from build123d import *

# Parameters (mm, degrees)
F0_R     = 22
F0_R_2   = 17.5
F0_R_3   = 12
F1_DEPTH = 8
F2_DEPTH = 20
F3_R     = 3
F4_R     = 1
F5_R     = 1


with BuildPart() as f1:
    # F0 (on Front) → F1 (new body)
    with BuildSketch(Plane.XZ):
        Circle(F0_R)
        Circle(F0_R_2, mode=Mode.SUBTRACT)
        Circle(F0_R_2)
        Circle(F0_R_3, mode=Mode.SUBTRACT)
    extrude(amount=F1_DEPTH)

    # F0 (on Front) → F2 (join)
    with BuildSketch(Plane.XZ):
        Circle(F0_R_2)
        Circle(F0_R_3, mode=Mode.SUBTRACT)
    extrude(amount=F2_DEPTH)

    # F3
    f3_edges = [f1.edges().sort_by_distance(p)[0] for p in [
        (-22, 0, 0),
    ]]
    fillet(f3_edges, radius=F3_R)

    # F4
    f4_edges = [f1.edges().sort_by_distance(p)[0] for p in [
        (-22, -8, 0),
    ]]
    fillet(f4_edges, radius=F4_R)

    # F5
    f5_edges = [f1.edges().sort_by_distance(p)[0] for p in [
        (-17.5, -20, 0),
    ]]
    fillet(f5_edges, radius=F5_R)


solid = f1.part
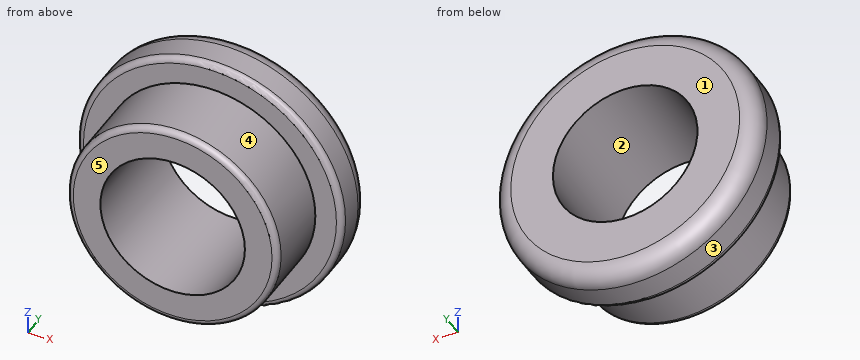
Source: CAD feature listing. Evaluate the final solid. Frame: model axes, mm. Face numbers are marked on the shaded views. A direction names the side the tool comes from. Round coordinates to 2 decimals unless told otherwise and drop trailing zeros. Loops run counter-clockwise (first coordinate to the right, second up) from the corner with the lowest first, then second, coordinate; pieces in that order, holes last. Notation, with made-up numbers: (76, 11.25) - (93, 11.25) arc R15 ccw to (93, 33.25) - close; hole circle Ø9 at (9.5, -28.5). An arc over 180 degrees is marked (long way). Write item = value, one per line. Start each with the question number.
Item 1: Section query B-B on x = 0. Output: boundary loops of the cut face in (y, z).
Item 2: First-contact query: pin 1 Ø5 at (x, z) = (-16, 5.5) entering from +Y; pin 2 Ø1.5 at (x, y) = (10.5, -5) entering from +Z; pin 3 Ø6 at (x, y) = (-10, -16) entering from -Z; pin 4 Ø2 at (x, y) = (-10, -9.5) entering from +Z. Flat tips, straight axial feed; report the tip coordinate or a pass-through.
Item 3: Section query C-C on y = -15.25. Output: boundary loops of the cut face in (x, z), plus the area to 3 significant figures.
Item 4: Section query A-A on z = 0. Output: boundary loops of the cut face in (x, y), plus the area to 3 significant figures.
Item 5: Mould query, pull axis Z, two halves, no side actions, for the marked faces 1, 2 and 3. Classes: released by +Z, released by -Z, zero draft, split by the parting line, or undercut.
Item 6: Reachability of the marked faces 4 and 5 from +Z, -Z, +X, -X, +Y, -Y: full face, straight path, thin tool, end or side. Return the list, or none.
Item 7: Material intervals for line 1 (X direction, y = -13, z = -0.5); line 2 (Z direction, x = 0, y = -4.5); line 3 (Z direction, x = 0, y = -16), sorted ascending.
Results list:
q1.outline = (-20, -16.5) arc R1 ccw to (-19, -17.5) - (-8, -17.5) - (-8, -21) arc R1 ccw to (-7, -22) - (-3, -22) arc R3 ccw to (0, -19) - (0, -12) - (-20, -12) - close; (-20, 12) - (0, 12) - (0, 19) arc R3 ccw to (-3, 22) - (-7, 22) arc R1 ccw to (-8, 21) - (-8, 17.5) - (-19, 17.5) arc R1 ccw to (-20, 16.5) - close
q2.pin_1 = 0
q2.pin_2 = 19.72
q2.pin_3 = -16.04
q2.pin_4 = 15.01
q3.outline = circle Ø35 at (0, 0); hole circle Ø24 at (0, 0)
q3.area = 510 mm²
q4.outline = (-22, -7) arc R1 ccw to (-21, -8) - (-17.5, -8) - (-17.5, -19) arc R1 ccw to (-16.5, -20) - (-12, -20) - (-12, 0) - (-19, 0) arc R3 ccw to (-22, -3) - close; (12, -20) - (16.5, -20) arc R1 ccw to (17.5, -19) - (17.5, -8) - (21, -8) arc R1 ccw to (22, -7) - (22, -3) arc R3 ccw to (19, 0) - (12, 0) - close
q4.area = 287 mm²
q5.face_1 = zero draft
q5.face_2 = undercut
q5.face_3 = split by the parting line
q6.face_4 = -Y
q6.face_5 = +Z, -Z, +X, -X, -Y
q7.line_1 = -17.49 to -11.99, 11.99 to 17.49
q7.line_2 = -22 to -12, 12 to 22
q7.line_3 = -17.5 to -12, 12 to 17.5
